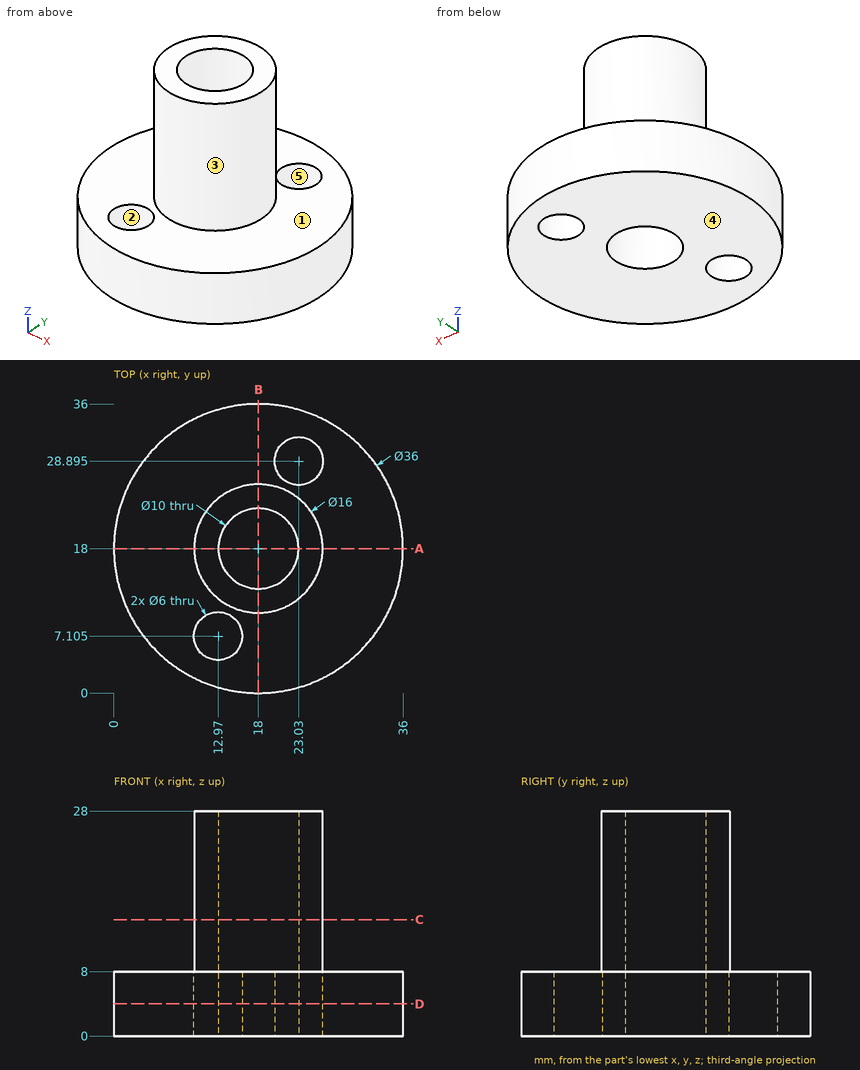
Here's the drawing with two shaded views (mm, measured from the low corner). I have some questions. A direction names the side the tool comes from. Give positions to 0.01 mm unless a question says otherwise; leave off trailing zeros. Order: outer loops, then holes, each group sorted by start corner. A loop starts at its lowest first (then second) coordinate and runs counter-clockwise, first axis right, second up.
Q1. Suppose I cut it at A-A, the plane y = 18. Write out the boundary of the cut face in (x, z).
Q2. I'm going to push flat-ended pins straight in: P1, Ø4, axis at x = 7.5, y = 10, coming from the +Z side; P2, Ø6, axis at x = 18, y = 18, coming from the -Z side; P3, Ø8, axis at x = 18.5, z = 23.5, coming from the -Y side. Where does each tip first touch, or does it pass through?
Q3. Suppose I cut it at D-D, the plane z = 4. Write out the boundary of the cut face in (x, y) (1 decimal).
Q4. We'd pull the mould along X, two halves only. Please class the marked faces 3, 4 and 5: +X half, -X half, draft (parallel to the pull), parting line (faces both ways), or undercut.
Q5. If I drill on line 1 along Y through (x, z) = (18, 14.75); line 2 along Y through (x, z) = (21.5, 6.25) (1 decimal); line 3 along Z through (x, y) = (26.5, 27), over which ranges is the centre line in solid material (lowest first)?
Q6. For the marked faces 1 and 2, which set-ups out of +Z, -Z, +X, -X, +Y, -Y let a thin tool reach every point of the face, with its end or its side?
Q7. Suppose I cut it at C-C, the plane z = 14.5. Write out the boundary of the cut face in (x, y).
Solution:
1. outline: (0, 0) - (13, 0) - (13, 28) - (10, 28) - (10, 8) - (0, 8) - close; (23, 0) - (36, 0) - (36, 8) - (26, 8) - (26, 28) - (23, 28) - close
2. P1: stops at z = 8
2. P2: passes through
2. P3: stops at y = 10
3. outline: circle Ø36 at (18, 18); hole circle Ø6 at (13, 7.1); hole circle Ø10 at (18, 18); hole circle Ø6 at (23, 28.9)
4. face 3: parting line
4. face 4: draft
4. face 5: undercut
5. line 1: y = 10 to 13, 23 to 26
5. line 2: y = 0.3 to 14.4, 21.6 to 26.3, 31.5 to 35.7
5. line 3: z = 0 to 8
6. face 1: +Z
6. face 2: +Z, -Z
7. outline: circle Ø16 at (18, 18); hole circle Ø10 at (18, 18)
